Autodesk Inventor part; units mm, degrees
ref_plane "YZ Plane" through (0, 0, 0) normal (1, 0, 0) x (0, 1, 0)
ref_plane "XZ Plane" through (0, 0, 0) normal (0, 1, 0) x (-1, 0, 0)
ref_plane "XY Plane" through (0, 0, 0) normal (0, 0, 1) x (1, 0, 0)
sketch "Skizze1" plane through (0, 0, 0) normal (0, 1, 0) x (-1, 0, 0)
  line L0 (-4.6, 12.6) -> (-4.6, 0)
  arc A0 (-4.6, 0) -> (0, -4.6) centre (0, 0) ccw
  line L1 (0, -4.6) -> (12.6, -4.6)
  arc A1 (12.6, -4.6) -> (17.2, 0) centre (12.6, 0) ccw
  line L2 (17.2, 0) -> (0, 0)
  line L3 (0, 0) -> (0, 17.2)
  arc A2 (0, 17.2) -> (-4.6, 12.6) centre (0, 12.6) ccw
  point P0 (0, 0)
  dimension "d0" = 4.6
  dimension "d1" = 21.8
extrude "Extrusion1" add sketch "Skizze1" along normal blind 197.2
sketch "Skizze2" plane through (0, 0, -4.6) normal (0, 0, -1) x (-1, 0, 0)
  line L0 (-4.6, 0) -> (17.2, 21.8)
  line L1 (17.2, 0) -> (17.2, 197.2)
  line L2 (17.2, 0) -> (12.6, 0)
  line L3 (17.2, 21.8) -> (17.2, 0)
  line L4 (17.2, 0) -> (-4.6, 0)
  line L5 (17.2, 197.2) -> (-4.6, 197.2)
  line L6 (-4.6, 197.2) -> (17.2, 175.4)
  line L7 (17.2, 197.2) -> (17.2, 175.4)
  point P0 (0, 0)
  dimension "d4" = 45
  dimension "d7" = 45
extrude "Extrusion2" cut sketch "Skizze2" against normal through all
sketch "Skizze3" plane through (4.6, 0, 0) normal (1, 0, 0) x (0, 0, -1)
  line L0 (4.6, 0) -> (-17.2, 21.8)
  line L1 (-17.2, 4.6) -> (-17.2, 192.6)
  line L2 (-17.2, 21.8) -> (-17.2, 0)
  line L3 (-17.2, 0) -> (4.6, 0)
  line L4 (-17.2, 175.4) -> (-17.2, 197.2)
  line L5 (-17.2, 197.2) -> (4.6, 197.2)
  line L6 (4.6, 197.2) -> (-17.2, 175.4)
  point P0 (0, 0)
  point P1 (4.6, 4.6)
  point P2 (-12.6, 197.2)
  dimension "d8" = 45
  dimension "d9" = 45
extrude "Extrusion3" cut sketch "Skizze3" against normal through all
properties part number "winkelTop" material "Kiefer"
Here's how the part is built. I have some questions about the finished solid (model axes, mm). A direction names the side the tool comes from. Coordinates: 2 decimals unless noted, no trailing zeros. Order: outer loops, then holes, each group sorted by start corner. A loop starts at its lowest first (then second) coordinate and runs counter-clockwise, first axis right, second up. Notation, with made-up numbers: (79, 44) - (106, 44) arc R18 cw to (106, 66) - close; hole circle Ø9 at (16, -32). An arc over 180 degrees is marked (long way). One line per question, with ' | ' between items. Start each with the question number.
1. If we section it at C-C (x = -15.25): Write out the boundary of the cut face in (y, z), and give its area (3 significant figures).
2. If we section it at A-A (y = 61): Write out the boundary of the cut face in (x, z), and give its area (3 significant figures).
3. Which directions (+Z, -Z, +X, -X, +Y, -Y) give clear straight access to the entire face, cutting with the end or side of a thin tool? Please do faces 1 (the flat face through (0, 97, 8)), 2 (the cylindrical face through (3.288, 97.46, 15.817)).
4. I'm going to push flat-ended pins straight in: pin 1 Ø10 at (x, y) = (-10, 82) entering from +Z; pin 2 Ø1 at (x, z) = (1, 1) entering from +Y; pin 3 Ø3 at (y, z) = (135, 12) entering from -X. Where does each tip first touch, or does it pass through?
5. If we section it at B-B (z = 5): Write out the boundary of the cut face in (x, y), and give its area (3 significant figures).
6. Please list where these lines run through material, in increasing order: line 1 along X through (y, z) = (155, 4); line 2 along Z through (x, y) = (-11, 170.5); line 3 along Z through (x, y) = (3.25, 85.5). Write a range as [from, to].
Model answer:
1) outline: (19.85, -3.76) - (177.35, -3.76) - (177.35, 0) - (19.85, 0) - close | area: 592 mm²
2) outline: (-17.2, 0) arc R4.6 ccw to (-12.6, -4.6) - (0, -4.6) arc R4.6 ccw to (4.6, 0) - (4.6, 12.6) arc R4.6 ccw to (0, 17.2) - (0, 0) - close | area: 166 mm²
3) face 1: +Z, -X, +Y, -Y | face 2: +Z, +X, +Y, -Y
4) pin 1: stops at z = 0 | pin 2: stops at y = 192.1 | pin 3: stops at x = 0
5) outline: (0, 9.6) - (4.6, 9.6) - (4.6, 187.6) - (0, 187.6) - close | area: 819 mm²
6) line 1: x = [0, 4.6] | line 2: z = [-4.6, 0] | line 3: z = [-3.26, 15.86]
